The listing builds one solid part. Answer for the finished solid, in the listing's coordinates (mm). Face numbers are marked on the shaded views. A direction names the side the tool comes from. Round coordinates to 2 decimals unless told otherwise and drop trailing zeros. Write each loop counter-clockwise with the first axis right and the second up, starting at its lowest first coordinate (ties: lowest second). Pieces come first, ordered by that corner, then holes. Notation, with made-up numbers: M -19,-38.75 L -7,-38.75 A17 ccw -7,-13.75 Z; hole C -33,-24.75 d1. An arc over 180 degrees is marked long. Write each question's results on one line, items separated by ' | '.
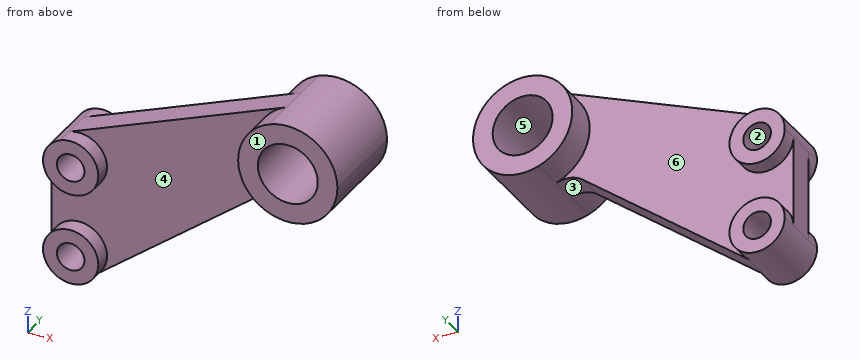
from build123d import *

# Parameters (mm, degrees)
F0_R     = 13.0048
F1_DEPTH = 20.0025
F2_DEPTH = 5.9944
F0_R_2   = 5.9944
F3_DEPTH = 13.0048


with BuildPart() as f1:
    # F0 (on Front) → F1 (new body, symmetric)
    with BuildSketch(Plane.XZ):
        with BuildLine():
            ThreePointArc((-7.110495, -20.331699), (12.465608, -17.56547), (21.5392, 0))
            ThreePointArc((21.5392, 0), (11.988357, 17.894593), (-8.194164, 19.919659))
            ThreePointArc((-8.194164, 19.919659), (-21.531398, -0.57968), (-7.110495, -20.331699))
        make_face()
        Circle(F0_R, mode=Mode.SUBTRACT)
    extrude(amount=F1_DEPTH, both=True)

    # F0 (on Front) → F2 (join, symmetric)
    with BuildSketch(Plane.XZ):
        with BuildLine():
            ThreePointArc((-7.110495, -20.331699), (-21.531398, -0.57968), (-8.194164, 19.919659))
            Line((-8.194164, 19.919659), (-102.558934, -18.898298))
            ThreePointArc((-102.558934, -18.898298), (-91.313367, -20.026651), (-85.9917, -29.9974))
            ThreePointArc((-85.9917, -29.9974), (-97.9932, -41.9989), (-109.9947, -29.9974))
            Line((-109.9947, -29.9974), (-109.9947, -70.0024))
            ThreePointArc((-109.9947, -70.0024), (-97.9932, -58.0009), (-85.9917, -70.0024))
            ThreePointArc((-85.9917, -70.0024), (-87.186467, -75.222604), (-90.532888, -79.40345))
            Line((-90.532888, -79.40345), (-18.520641, -22.257298))
            ThreePointArc((-18.520641, -22.257298), (-13.063266, -19.826762), (-7.110495, -20.331699))
        make_face()
    extrude(amount=F2_DEPTH, both=True)

    # F0 (on Front) → F3 (join, symmetric)
    with BuildSketch(Plane.XZ):
        with BuildLine():
            ThreePointArc((-109.9947, -70.0024), (-103.213404, -80.809133), (-90.532888, -79.40345))
            ThreePointArc((-90.532888, -79.40345), (-87.186467, -75.222604), (-85.9917, -70.0024))
            ThreePointArc((-85.9917, -70.0024), (-97.9932, -58.0009), (-109.9947, -70.0024))
        make_face()
        with Locations((-97.9932, -70.0024)):
            Circle(F0_R_2, mode=Mode.SUBTRACT)
        with BuildLine():
            ThreePointArc((-85.9917, -29.9974), (-91.313367, -20.026651), (-102.558934, -18.898298))
            ThreePointArc((-102.558934, -18.898298), (-107.963949, -23.317567), (-109.9947, -29.9974))
            ThreePointArc((-109.9947, -29.9974), (-97.9932, -41.9989), (-85.9917, -29.9974))
        make_face()
        with Locations((-97.9932, -29.9974)):
            Circle(F0_R_2, mode=Mode.SUBTRACT)
    extrude(amount=F3_DEPTH, both=True)


solid = f1.part
1) Section B-B (x = 0) is taken. Determine the outline of the cut face in (y, z).
Return value:
outline: M -20,-21.54 L 20,-21.54 L 20,-13 L -20,-13 Z; M -20,13 L 20,13 L 20,21.54 L -20,21.54 Z
2) The mould has two halves that part along Z. Classify the marked faces 1, 2 and 3: +Z half, -Z half, draft (parallel to the pull), parting line (faces both ways), or undercut.
Return value:
face 1: draft | face 2: undercut | face 3: -Z half
3) Find the intervals of material crossed by line 1 (Z direction, x = 0, y = -10); line 2 (Z direction, x = -101.5, y = -5); line 3 (Y direction, x = -89, z = -15), in increasing order.
Return value:
line 1: -21.54 to -13, 13 to 21.54 | line 2: -81.48 to -74.86, -65.14 to -34.86, -25.14 to -18.46 | line 3: -5.99 to 5.99
4) Section A-A (y = 11) is taken. Determine the outline of the cut face in (x, z).
Return value:
outline: M -109.99,-30 A12 ccw long -102.56,-18.9 A12 ccw Z; M -90.53,-79.4 A12 ccw -85.99,-70 A12 ccw long Z; C 0,0 d43.08; hole C -97.99,-70 d11.99; hole C -97.99,-30 d11.99; hole C 0,0 d26.01
5) Section D-D (y = -17) is taken. Determine the outline of the cut face in (x, z).
Return value:
outline: C 0,0 d43.08; hole C 0,0 d26.01
6) Each of these flat-tipped pins is pushed along its axis until it touches: pin 1 (19 mm diameter, centred on x = -96, z = -27.5, fed in from +Y); pin 2 (1 mm diameter, centred on y = -9.5, z = -69, fed in from +X); pin 3 (7 mm diameter, centred on x = -94, z = -24, fed in from -Y); pin 4 (15.5 mm diameter, centred on x = 0, z = 0, fed in from +Y). Where does it stop, or does it pass through?
Return value:
pin 1: y = 13 | pin 2: x = -86 | pin 3: y = -13 | pin 4: through
7) Section C-C (z = -26) is taken. Determine the outline of the cut face in (x, y), then the cut area to 3 significant figures.
Return value:
outline: M -109.31,-13 L -102.46,-13 L -102.46,13 L -109.31,13 Z; M -93.53,-13 L -86.68,-13 L -86.68,-5.99 L -23.24,-5.99 L -23.24,5.99 L -86.68,5.99 L -86.68,13 L -93.53,13 Z | area: 1,120 mm²
8) A tool of negligible diameter and unlimited length cuts with its end or side. For the marked faces 4, 5 and 6, from which of +Z, -Z, +X, -X, +Y, -Y can it reach the whole face along a straight path? Write none if from no direction.
Return value:
face 4: -Y | face 5: +Y, -Y | face 6: +Y
